Part model, mm, in its own coordinate system. Coordinates: 2 decimals unless noted, no trailing zeros. Loops run counter-clockwise (first coordinate to the right, second up) from the corner with the lowest first, then second, coordinate; pieces in that order, holes last. Notation, with made-up numbers: M 54.5,52.5 L 95.5,52.5 A22 cw 95.5,77.5 Z; hole C 21.25,58.25 d3. An arc over 180 degrees is marked long. Answer as a JSON object with one key per item and string values. Group by question number.
1. Drop flat-ended pins along their axis: pin 1 Ø2 at (y, z) = (-49.5, 392) entering from +X; pin 2 Ø1.5 at (x, z) = (119.5, 393) entering from -Y. Give the stop position or say it passes through.
2. Drill centre lines: L1, parallel to X at y = -10, z = 393.5; L2, parallel to X at y = -36, z = 390.15; L3, parallel to Y at x = 131, z = 392.6. Where is each one in solid material? Low to high.
3. Mould opens along Y. For faces 1 (the face through (68.989, -36.225, 391.427)), 2 (the face through (132.52, -29.87, 391.43)) say: released by +Y, released by -Y, zero draft, split by the parting line, or undercut.
4. Saw through at A-A on x = 130. Write the cut outline in (y, z), then the cut area to 3 significant figures.
5. Saw through at D-D on y = -63. Write the cut outline in (x, z).
6. Saw through at B-B on y = -24.5. Write the cut outline in (x, z).
Autodesk Inventor part; units mm, degrees
ref_plane "РабПлоскость1" through (67.2056, 19.9956, 394.3851) normal (0, 0, -1) x (-0.9999, -0.0165, 0)
ref_plane "YZ Plane" through (0, 0, 0) normal (1, 0, 0) x (0, 1, 0)
ref_plane "XZ Plane" through (0, 0, 0) normal (0, 1, 0) x (-1, 0, 0)
ref_plane "РабПлоскость1" through (67.2056, 19.9956, 394.3851) normal (0, 0, -1) x (-0.9999, -0.0165, 0)
sketch "Эскиз1" plane through (67.2056, 19.9956, 394.3851) normal (0, 0, -1) x (-0.9999, -0.0165, 0)
  line L0 (-9.6218, -57.1442) -> (-3, -57.1442)
  arc A0 (-9.6218, -57.1442) -> (-12.6119, -59.9009) centre (-9.6218, -60.1442) ccw
  arc A1 (-3, -57.1442) -> (0, -54.1442) centre (-3, -54.1442) ccw
  line L1 (0, -54.1442) -> (0, 5.8558)
  line L2 (0, 5.8558) -> (-13.2857, 5.8558)
  line L3 (-13.2857, -0.1442) -> (-13.2857, 5.8558)
  line L4 (-13.2857, -0.1442) -> (-26.5714, -0.1442)
  line L5 (-26.5714, -0.1442) -> (-26.5714, 5.8558)
  line L6 (-26.5714, 5.8558) -> (-39.8571, 5.8558)
  line L7 (-39.8571, -0.1442) -> (-39.8571, 5.8558)
  line L8 (-39.8571, -0.1442) -> (-53.1429, -0.1442)
  line L9 (-53.1429, -0.1442) -> (-53.1429, 5.8558)
  line L10 (-53.1429, 5.8558) -> (-66.4286, 5.8558)
  line L11 (-66.4286, -0.1442) -> (-66.4286, 5.8558)
  line L12 (-66.4286, -0.1442) -> (-79.7143, -0.1442)
  line L13 (-79.7143, -0.1442) -> (-79.7143, 5.8558)
  line L14 (-79.7143, 5.8558) -> (-93, 5.8558)
  line L15 (-93, 5.8558) -> (-93, -54.1442)
  arc A2 (-93, -54.1442) -> (-90, -57.1442) centre (-90, -54.1442) ccw
  line L16 (-90, -57.1442) -> (-83.3782, -57.1442)
  arc A3 (-80.3881, -59.9009) -> (-83.3782, -57.1442) centre (-83.3782, -60.1442) ccw
  arc A4 (-80.3881, -59.9009) -> (-12.6119, -59.9009) centre (-46.5, -57.1442) ccw
  circle A5 centre (-46.5, -50.1442) radius 18
  line L17 (-74.5714, -0.1442) -> (-79.7143, -0.1442)
  line L18 (-21.4286, -0.1442) -> (-26.5714, -0.1442)
  line L19 (-49.5, -0.1442) -> (-53.1429, -0.1442)
  circle A6 centre (-46.5, -50.1442) radius 18 construction
  point P0 (67.5262, -18.8845)
  dimension "d0" = 6
extrude "Выдавливание1" add sketch "Эскиз1" along normal blind 6
sketch "Эскиз2" plane through (67.2056, 19.9956, 388.3851) normal (0, 0, -1) x (-0.9999, -0.0165, 0)
  circle A0 centre (-46.5, -15.5) radius 1.5
  line L0 (-49.5, -10.3334) -> (-49.5, -0.1442) construction
  line L1 (-43.5, -0.1442) -> (-43.5, -10.3334) construction
  line L2 (-43.5, -20.6667) -> (-43.5, -31) construction
  line L3 (-49.5, -31) -> (-49.5, -20.6667) construction
  line L4 (-49.5, -31) -> (-43.5, -31)
  line L5 (-43.5, -31) -> (-43.5, -20.6667)
  line L6 (-43.5, -20.6667) -> (-49.5, -20.6667)
  line L7 (-49.5, -20.6667) -> (-49.5, -31)
  line L8 (-49.5, -10.3334) -> (-43.5, -10.3334)
  line L9 (-43.5, -10.3334) -> (-43.5, -0.1442)
  line L10 (-43.5, -0.1442) -> (-49.5, -0.1442)
  line L11 (-49.5, -0.1442) -> (-49.5, -10.3334)
  line L12 (-17.1786, -8.65) -> (-17.1786, -6.35)
  line L13 (-17.1786, -6.35) -> (-18.4286, -6.35)
  line L14 (-18.4286, -6.35) -> (-18.4286, -0.1442)
  line L15 (-21.4286, -0.1442) -> (-21.4286, -6.35)
  line L16 (-21.4286, -6.35) -> (-22.6786, -6.35)
  line L17 (-22.6786, -6.35) -> (-22.6786, -8.65)
  line L18 (-22.6786, -8.65) -> (-21.4286, -8.65)
  line L19 (-21.4286, -8.65) -> (-21.4286, -15)
  line L20 (-21.4286, -15) -> (-18.4286, -15)
  line L21 (-18.4286, -15) -> (-18.4286, -8.65)
  line L22 (-18.4286, -8.65) -> (-17.1786, -8.65)
  line L23 (-21.4286, -0.1442) -> (-18.4286, -0.1442)
  line L24 (-46.5, -10.3334) -> (-46.5, -0.1442) construction
  line L25 (-75.8214, -8.65) -> (-75.8214, -6.35)
  line L26 (-75.8214, -6.35) -> (-74.5714, -6.35)
  line L27 (-74.5714, -6.35) -> (-74.5714, -0.1442)
  line L28 (-71.5714, -0.1442) -> (-71.5714, -6.35)
  line L29 (-71.5714, -6.35) -> (-70.3214, -6.35)
  line L30 (-70.3214, -6.35) -> (-70.3214, -8.65)
  line L31 (-70.3214, -8.65) -> (-71.5714, -8.65)
  line L32 (-71.5714, -8.65) -> (-71.5714, -15)
  line L33 (-71.5714, -15) -> (-74.5714, -15)
  line L34 (-74.5714, -15) -> (-74.5714, -8.65)
  line L35 (-74.5714, -8.65) -> (-75.8214, -8.65)
  line L36 (-71.5714, -0.1442) -> (-74.5714, -0.1442)
  point P0 (67.5262, -18.8845)
extrude "Выдавливание2" cut sketch "Эскиз2" against normal blind 6
equation "\"d1\" = d0"
equation "\"d3\" = d0"
properties part number "motor2"
Outcome:
{
 "1": {"pin 1": "stops at x = 146.41", "pin 2": "stops at y = -70.12"},
 "2": {"L1": "x = 67.7 to 111.21, 117.21 to 160.71", "L2": "x = 68.78 to 97.79, 131.26 to 150.4", "L3": "y = -66.18 to -36.63, -22.12 to 26.9"},
 "3": {"face 1": "released by -Y", "face 2": "undercut"},
 "4": {"outline": "M -66.71,388.39 L -38.57,388.39 L -38.57,394.39 L -66.71,394.39 Z; M -20.18,388.39 L 26.89,388.39 L 26.89,394.39 L -20.18,394.39 Z", "area": "451 mm²"},
 "5": {"outline": "M 93.5,388.39 L 135.79,388.39 L 135.79,394.39 L 93.5,394.39 Z"},
 "6": {"outline": "M 67.94,388.39 L 97.2,388.39 L 97.2,394.39 L 67.94,394.39 Z; M 131.85,388.39 L 160.95,388.39 L 160.95,394.39 L 131.85,394.39 Z"}
}
